The listing builds one solid part. Answer for the finished solid, in the listing's coordinates (mm). A direction names the side the tool comes from. Coordinates: 2 decimals unless noted, no trailing zeros. Write each loop counter-clockwise with the first axis right and the second up, starting at its lowest first coordinate (ties: lowest second). Pieces come first, ordered by that corner, then holes.
from build123d import *

# Parameters (mm, degrees)
SKETCH1_R           = 20
BOSS_EXTRUDE1_DEPTH = 5
SKETCH1_3_R         = 20
SKETCH1_3_R_2       = 17.5
BOSS_EXTRUDE3_DEPTH = 7
SKETCH3_R           = 7.5
CUT_EXTRUDE2_DEPTH  = 7


with BuildPart() as part:
    # Sketch1 → Boss-Extrude1 (new body)
    with BuildSketch(Plane(origin=(0, 0, 0), x_dir=(1, 0, 0), z_dir=(0, 1, 0))):
        with Locations(Location((0, 0, 0), (0, 0, 270))):
            Circle(SKETCH1_R)
    extrude(amount=BOSS_EXTRUDE1_DEPTH)

    # Sketch1_3 → Boss-Extrude3 (add)
    with BuildSketch(Plane(origin=(0, 0, 0), x_dir=(1, 0, 0), z_dir=(0, 1, 0))):
        with Locations(Location((0, 0, 0), (0, 0, 270))):
            Circle(SKETCH1_3_R)
        with Locations(Location((0, 0, 0), (0, 0, 270))):
            Circle(SKETCH1_3_R_2, mode=Mode.SUBTRACT)
    extrude(amount=BOSS_EXTRUDE3_DEPTH)

    # Sketch3 → Cut-Extrude2 (cut)
    with BuildSketch(Plane(origin=(0, 5, 0), x_dir=(1, 0, 0), z_dir=(0, 1, 0))):
        with Locations(Location((0, 0, 0), (0, 0, 270))):
            Circle(SKETCH3_R)
    extrude(amount=-CUT_EXTRUDE2_DEPTH, mode=Mode.SUBTRACT)


solid = part.part
1. Section A-A on z = 0 is taken. Give the vertices of the cut face in (x, y).
Results found:
outline: (-20, 0) - (-7.5, 0) - (-7.5, 5) - (-17.5, 5) - (-17.5, 7) - (-20, 7) - close; (7.5, 0) - (20, 0) - (20, 7) - (17.5, 7) - (17.5, 5) - (7.5, 5) - close
2. Section D-D on y = 0.5 is taken. Give the vertices of the cut face in (x, z), then the cut area to 3 significant figures.
Results found:
outline: circle Ø40 at (0, 0); hole circle Ø15 at (0, 0)
area: 1,080 mm2
3. Find the intervals of material crossed by L1, parallel to X at y = 1.65, z = 0; L2, parallel to X at y = 6.4, z = 0; L3, parallel to Y at x = -2.5, z = -12, in increasing order.
Results found:
L1: x = -20 to -7.5, 7.5 to 20
L2: x = -20 to -17.5, 17.5 to 20
L3: y = 0 to 5
4. Section B-B on x = 0 is taken. Give the vertices of the cut face in (y, z).
Results found:
outline: (0, -20) - (7, -20) - (7, -17.5) - (5, -17.5) - (5, -7.5) - (0, -7.5) - close; (0, 7.5) - (5, 7.5) - (5, 17.5) - (7, 17.5) - (7, 20) - (0, 20) - close
5. Section C-C on z = -15 is taken. Give the vertices of the cut face in (x, y).
Results found:
outline: (-13.23, 0) - (13.23, 0) - (13.23, 7) - (9.01, 7) - (9.01, 5) - (-9.01, 5) - (-9.01, 7) - (-13.23, 7) - close
6. A tool of negligible diameter and unlimited length cuts with its end or side. For faces 1 (the flat face through (0, 0, 9)), 2 (the flat face through (-8, 5, 0)), from which of +Z, -Z, +X, -X, +Y, -Y can it reach the whole face along a straight path? Write none if from no direction.
Results found:
face 1: +Z, -Z, +X, -X, -Y
face 2: +Y
7. Flat-ended cylindrical pins translate along their axes: P1, Ø1, axis at y = 6, z = -10.5, coming from the +X side; P2, Ø2, axis at y = 4.5, z = -7, coming from the +X side; P3, Ø2, axis at y = 3.5, z = -2.5, coming from the -X side; P4, Ø9, axis at x = 0, z = 0, coming from the +Y side. Find the tip coordinate at first contact, or state that the pin passes through.
Results found:
P1: stops at x = 17.32
P2: stops at x = 19.08
P3: stops at x = -19.94
P4: passes through
8. For a pull along Z with two mould halves and no side action, classify faces 3 (the flat face through (-18, 7, 0)), 4 (the cylindrical face through (0.33, 2.535, -7.493)), 5 (the cylindrical face through (-10.648, 5.986, -13.887)), 6 (the cylindrical face through (-19.524, 3.451, -4.336)) as pulls with the +Z half, pulls with the -Z half, needs draft (parallel to the pull), parting line crosses it, or undercut.
Results found:
face 3: needs draft
face 4: undercut
face 5: undercut
face 6: parting line crosses it
